Read the model definition and answer for the solid it produces. Units are mm, in the model's axes. Face numbers are marked on the shaded views. A direction names the side the tool comes from. Give positions to 0.01 mm unless a question says otherwise; leave off trailing zeros. Loops run counter-clockwise (first coordinate to the right, second up) from the corner with the lowest first, then second, coordinate; pieces in that order, holes last.
(1) Find section A-A, the plane x = 0. Write down the section's boundary in (y, z), then the cut area to 3 significant figures.
(2) Find section C-C, the plane z = -6. Write down the section's boundary in (x, y), then the cut area to 3 significant figures.
(3) Which of the six approach directions +Z, -Z, +X, -X, +Y, -Y give full straight-line access (tool end or side, diameter ignored) to the marked faces 1 and 2?
(4) Find section D-D, the plane z = 3.5. Write down the section's boundary in (x, y), then the cut area to 3 significant figures.
(5) Each of these flat-tipped pins is pushed along its axis until it touches: P1, Ø6, axis at x = 8.5, y = 0.5, coming from the -Z side; P2, Ø9, axis at x = 0, y = 0, coming from the -Z side; P3, Ø3, axis at x = -3.5, z = 3.5, coming from the +Y side; P4, Ø4, axis at x = 3, y = -2.5, coming from the -Z side. Where does it stop, or does it pass through?
(6) Straight lines are drawn through the part: probe 1 along Y at (x, z) = (0, -0.5); probe 2 along Y at (x, z) = (-3.25, -1); probe 3 along X at (y, z) = (-1.25, 1.5). For each, find the intervals that lie inside material, in ascending order.
(7) Determine the mould class of the marked faces 3, 4 and 5 for opening direction Y: pulls with the +Y half, pulls with the -Y half, needs draft (parallel to the pull), parting line crosses it, or undercut.
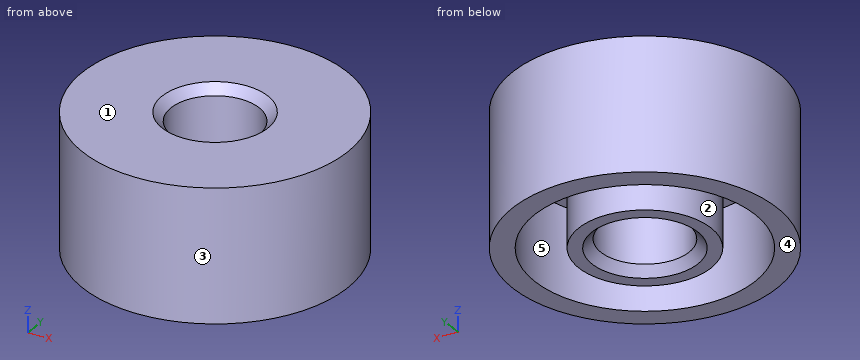
Autodesk Inventor part; units mm, degrees
ref_plane "YZ Plane" through (0, 0, 0) normal (1, 0, 0) x (0, 1, 0)
ref_plane "XZ Plane" through (0, 0, 0) normal (0, 1, 0) x (-1, 0, 0)
ref_plane "XY Plane" through (0, 0, 0) normal (0, 0, 1) x (1, 0, 0)
sketch "Skizze1" plane through (0, 0, 0) normal (0, 0, 1) x (1, 0, 0)
  circle A0 centre (0, 0) radius 15
  dimension "d0" = 30
extrude "Extrusion1" add sketch "Skizze1" along normal mid plane 15
sketch "Skizze2" plane through (0, 0, 7.5) normal (0, 0, 1) x (1, 0, 0)
  point P0 (0, 0)
  point P1 (0, 0)
hole "Bohrung1" at (0, 0, 7.5) direction (0, 0, -1) diameter 10 end through all
chamfer "Fasen1" distance 1 angle 45 2 edges at (0, 5, 7.5) (0, 5, -7.5)
sketch "Skizze3" plane through (0, 0, -7.5) normal (0, 0, -1) x (-1, 0, 0)
  circle A0 centre (0, 0) radius 12.5
  circle A1 centre (0, 0) radius 7.5
  dimension "d13" = 25
  dimension "d14" = 15
extrude "Extrusion2" cut sketch "Skizze3" against normal blind 10
equation "\"d0\" = Gleitbuchse_Aussendurchmesser"
equation "\"d1\" = Hoehe_Buchse"
equation "\"d3\" = Gleitbuchse_Innendurchmesser"
equation "\"d10\" = Fase"
equation "\"d13\" = Feder_aussen"
equation "\"d14\" = Feder_innen"
equation "\"d15\" = Federfuehrung_Tiefe"
equation "\"Gleitbuchse_Aussendurchmesser\" = 30"
equation "\"Gleitbuchse_Innendurchmesser\" = 10"
equation "\"Hoehe_Buchse\" = 15"
equation "\"Fase\" = 1"
equation "\"Federfuehrung_Tiefe\" = 10"
equation "\"Feder_aussen\" = 25"
equation "\"Feder_innen\" = 15"
properties part number "TS_Magazin_Gleitbuchse_int"
Entries:
1. outline: (-15, -7.5) - (-12.5, -7.5) - (-12.5, 2.5) - (-7.5, 2.5) - (-7.5, -7.5) - (-6, -7.5) - (-5, -6.5) - (-5, 6.5) - (-6, 7.5) - (-15, 7.5) - close; (5, -6.5) - (6, -7.5) - (7.5, -7.5) - (7.5, 2.5) - (12.5, 2.5) - (12.5, -7.5) - (15, -7.5) - (15, 7.5) - (6, 7.5) - (5, 6.5) - close
1. area: 198 mm2
2. outline: circle Ø30 at (0, 0); circle Ø15 at (0, 0); hole circle Ø25 at (0, 0); hole circle Ø10 at (0, 0)
2. area: 314 mm2
3. face 1: +Z, +X, -X, +Y, -Y
3. face 2: -Z
4. outline: circle Ø30 at (0, 0); hole circle Ø10 at (0, 0)
4. area: 628 mm2
5. P1: stops at z = -7.5
5. P2: passes through
5. P3: stops at y = 14.87
5. P4: stops at z = -7.41
6. probe 1: y = -15 to -12.5, -7.5 to -5, 5 to 7.5, 12.5 to 15
6. probe 2: y = -14.64 to -12.07, -6.76 to -3.8, 3.8 to 6.76, 12.07 to 14.64
6. probe 3: x = -14.95 to -12.44, -7.4 to -4.84, 4.84 to 7.4, 12.44 to 14.95
7. face 3: parting line crosses it
7. face 4: needs draft
7. face 5: undercut
